Geometry: final body of the model. Coordinates: model frame, mm. Face numbers are marked on the shaded views. A direction names the side the tool comes from. Round coordinates to 2 decimals unless told otherwise and drop trailing zeros. Loops run counter-clockwise (first coordinate to the right, second up) from the corner with the lowest first, then second, coordinate; pieces in that order, holes last. Notation, with made-up numbers: (36, -31) - (55, -31) arc R33 ccw to (55, -1) - close; hole circle Ø7 at (62.5, 82). An arc over 180 degrees is marked (long way). Write item = value, one per line. Start each with the question number.
Item 1: Section D-D (z = 2.9). Count the separate pieces of the cut face and the enclosed holes in it, plus the area to 3 significant figures.
Item 2: Section C-C (y = 24). Return loops of the section in (x, z).
Item 3: Draft query along X for the marked faces 1, 2 and 3. Return one class per face: pulls with the +X half, pulls with the -X half, needs draft (parallel to the pull), parting line crosses it, or undercut.
Item 4: Line query: line 1 (Y direction, x = -27, z = 2.3); line 2 (X direction, y = 27, z = 2.75); line 3 (X direction, y = 5, z = 3.25). Output: solid intervals per line, ascending. Write a range as from..to.
Item 5: Section B-B (y = 36.25). Return loops of the section in (x, z), plus the area to 3 significant figures.
Item 6: First-contact query: pin 1 (2 mm diameter, centred on y = 0, z = 1, fed in from -X); pin 2 (2.5 mm diameter, centred on x = -12, y = -6.25, fed in from +Z); pin 3 (1.2 mm diameter, centred on x = -27, z = 1.5, fed in from -Y). Flat tips, straight axial feed; report the tip coordinate or a pass-through.
Item 7: Section A-A (x = 27). Return loops of the section in (y, z).
Item 8: Access query for the marked faces 4, 5 and 6. Directions: +Z, -Z, +X, -X, +Y, -Y. A direction counts if a zero-diameter tool reaches every point of the face in a straight line with its end or side. Return the directions, or none.
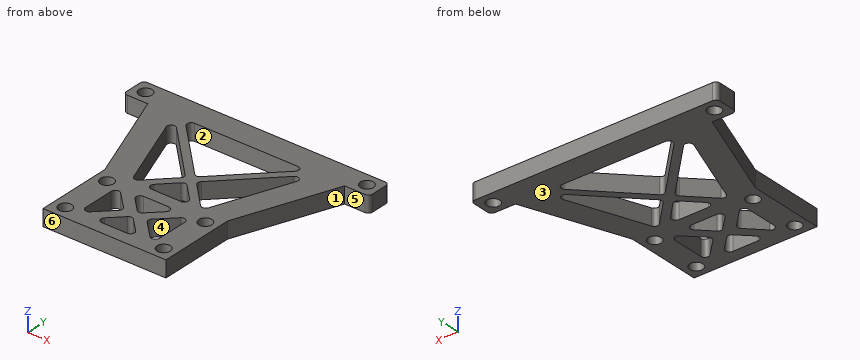
from build123d import *

# Parameters (mm, degrees)
F1_DEPTH = 4
F2_R     = 1.6
F3_DEPTH = 4
F5_DEPTH = 4
F6_R     = 1
F7_R     = 1
F9_DEPTH = 4
F10_R    = 1


with BuildPart() as f1:
    # F0 (on Top) → F1 (new body)
    with BuildSketch(Plane.XY):
        Polygon((-15, 9.25), (-15, -9.25), (15, -9.25), (15, 9.25), (24, 33.25), (30, 33.25), (30, 39.25), (-30, 39.25), (-30, 33.25), (-24, 33.25), align=None)
    extrude(amount=F1_DEPTH)

    # F2 (on face) → F3 (cut, through all)
    with BuildSketch(Plane.XY.offset(4)):
        with Locations((-12, 6.25)):
            Circle(F2_R)
        with Locations((12, 6.25)):
            Circle(F2_R)
        with Locations((-12, -6.25)):
            Circle(F2_R)
        with Locations((12, -6.25)):
            Circle(F2_R)
        with Locations((27, 36.25)):
            Circle(F2_R)
        with Locations((-27, 36.25)):
            Circle(F2_R)
    extrude(amount=-F3_DEPTH, mode=Mode.SUBTRACT)

    # F4 (on face) → F5 (cut, through all)
    with BuildSketch(Plane.XY.offset(4)):
        Polygon((-1.307755, 16.667609), (-17.591997, 33.25), (-8.591997, 9.25), align=None)
        Polygon((8.591997, 9.25), (17.591997, 33.25), (1.307755, 16.667609), align=None)
        Polygon((15, 33.25), (-15, 33.25), (0, 17.975365), align=None)
        Polygon((0, 15.359854), (-6, 9.25), (6, 9.25), align=None)
    extrude(amount=-F5_DEPTH, mode=Mode.SUBTRACT)

    # F6
    f6_edges = [f1.edges().sort_by_distance(p)[0] for p in [
        (17.591997, 33.25, 2),
        (15, 33.25, 2),
        (-15, 33.25, 2),
        (-17.591997, 33.25, 2),
        (0, 17.975365, 2),
        (8.591997, 9.25, 2),
        (-8.591997, 9.25, 2),
        (-6, 9.25, 2),
        (6, 9.25, 2),
        (0, 15.359854, 2),
        (-1.307755, 16.667609, 2),
        (1.307755, 16.667609, 2),
    ]]
    fillet(f6_edges, radius=F6_R)

    # F7
    f7_edges = [f1.edges().sort_by_distance(p)[0] for p in [
        (30, 39.25, 2),
        (30, 33.25, 2),
        (-30, 33.25, 2),
        (-30, 39.25, 2),
    ]]
    fillet(f7_edges, radius=F7_R)

    # F8 (on face) → F9 (cut, through all)
    with BuildSketch(Plane(origin=(0, 0, 0), x_dir=(1, 0, 0), z_dir=(0, 0, -1))):
        Polygon((-9, 6.25), (-9, -6.25), (-2.75, 0), align=None)
        Polygon((0, -0.744883), (-5.505117, -6.25), (5.505117, -6.25), align=None)
        Polygon((2.75, 0), (9, -6.25), (9, 6.25), align=None)
        Polygon((5.505117, 6.25), (-5.505117, 6.25), (0, 0.744883), align=None)
    extrude(amount=-F9_DEPTH, mode=Mode.SUBTRACT)

    # F10
    f10_edges = [f1.edges().sort_by_distance(p)[0] for p in [
        (-9, 6.25, 2),
        (-5.505117, 6.25, 2),
        (5.505117, 6.25, 2),
        (9, 6.25, 2),
        (-9, -6.25, 2),
        (-2.75, 0, 2),
        (5.505117, -6.25, 2),
        (9, -6.25, 2),
        (2.75, 0, 2),
        (0, -0.744883, 2),
        (-5.505117, -6.25, 2),
        (0, 0.744883, 2),
    ]]
    fillet(f10_edges, radius=F10_R)


solid = f1.part
Taken from the geometry:
q1.separate_pieces = 1
q1.enclosed_holes = 14
q1.area = 1,180 mm^2
q2.outline = (-20.53, 0) - (-14.12, 0) - (-14.12, 4) - (-20.53, 4) - close; (-8.51, 0) - (-5.92, 0) - (-5.92, 4) - (-8.51, 4) - close; (5.92, 0) - (8.51, 0) - (8.51, 4) - (5.92, 4) - close; (14.12, 0) - (20.53, 0) - (20.53, 4) - (14.12, 4) - close
q3.face_1 = pulls with the +X half
q3.face_2 = undercut
q3.face_3 = needs draft
q4.line_1 = 33.25..34.65, 37.85..39.25
q4.line_2 = -21.66..-15.25, -11.45..-8.86, 8.86..11.45, 15.25..21.66
q4.line_3 = -15..-13, -11..-4.06, 4.06..11, 13..15
q5.outline = (-30, 0) - (-28.6, 0) - (-28.6, 4) - (-30, 4) - close; (-25.4, 0) - (25.4, 0) - (25.4, 4) - (-25.4, 4) - close; (28.6, 0) - (30, 0) - (30, 4) - (28.6, 4) - close
q5.area = 214 mm^2
q6.pin_1 = -15
q6.pin_2 = through
q6.pin_3 = 33.25
q7.outline = (33.25, 0) - (34.65, 0) - (34.65, 4) - (33.25, 4) - close; (37.85, 0) - (39.25, 0) - (39.25, 4) - (37.85, 4) - close
q8.face_4 = +Z, -Z
q8.face_5 = +Z, -Z, +X, -Y
q8.face_6 = +Z, -Z, +X, -X, -Y
